Autodesk Inventor part; units mm, degrees
ref_plane "YZ Plane" through (0, 0, 0) normal (1, 0, 0) x (0, 1, 0)
ref_plane "XZ Plane" through (0, 0, 0) normal (0, 1, 0) x (-1, 0, 0)
ref_plane "XY Plane" through (0, 0, 0) normal (0, 0, 1) x (1, 0, 0)
sketch "Skizze1" plane through (0, 0, 0) normal (0, 1, 0) x (-1, 0, 0)
  line L0 (0, 0) -> (0, -54)
  line L1 (0, 0) -> (2, 0)
  line L2 (2, 0) -> (2, -10)
  line L3 (2, -10) -> (2.5, -10)
  line L4 (2.5, -10) -> (2.5, -40)
  line L5 (2.5, -40) -> (4, -40)
  line L6 (4, -40) -> (4, -44)
  line L7 (4, -44) -> (6, -44)
  line L8 (6, -44) -> (6, -48)
  line L9 (6, -48) -> (2.5, -48)
  line L10 (2.5, -48) -> (2.5, -46)
  line L11 (2.5, -46) -> (2, -46)
  line L12 (2, -46) -> (2, -54)
  line L13 (2, -54) -> (0, -54)
  point P0 (0, -27)
  point P1 (4.25, -48)
  point P2 (3.25, -40)
  point P3 (1, -54)
  point P4 (1, 0)
  dimension "d0" = 54
  dimension "d1" = 36
  dimension "d2" = 4
  dimension "d3" = 4
  dimension "d4" = 4
  dimension "d5" = 12
  dimension "d6" = 5
  dimension "d7" = 8
  dimension "d8" = 8
  dimension "d11" = 10
  dimension "d12" = 6
revolve "Umdrehung1" add sketch "Skizze1" angle 360 about axis through (0, 0, 0) along (0, 0, -1)
thread "Gewinde1"
chamfer "Fasen1" distance 0.5 angle 45 1 edges at (6, 0, -48)
chamfer "Fasen2" distance 0.5 angle 45 1 edges at (6, 0, -44)
sketch "Skizze2" plane through (0, 0, 0) normal (0, 0, 1) x (1, 0, 0)
  circle A0 centre (0, 0) radius 2
hole "Bohrung1" at (0, 0, 0) direction (0, 0, -1) diameter 3 end through all
properties part number "BRS"
Source: CAD feature listing. Evaluate the final solid. Frame: model axes, mm. A direction names the side the tool comes from. Give positions to 0.01 mm unless a question says otherwise; leave off trailing zeros. Order: outer loops, then holes, each group sorted by start corner. A loop starts at its lowest first (then second) coordinate and runs counter-clockwise, first axis right, second up. Notation, with made-up numbers: (46.5, 46.5) -> (91.5, 46.5) arc R22 ccw to (91.5, 52.5) -> close; hole circle Ø8 at (29, 5). An arc over 180 degrees is marked (long way). Use a Markdown table: item, result.
Q1. Pull-direction query (Y, two-part tool) for faces 4 (the face through (1, 2, -46)), 5 (the face through (4, -2, -44)), 6 (the face through (6, 0, -46)); classes: +Y half, -Y half, draft (parallel to the pull), parting line (faces both ways), or undercut.
A:
| item | result |
|---|---|
| face 4 | undercut |
| face 5 | draft |
| face 6 | parting line |
Q2. First-contact query: P1, Ø4, axis at y = 3.5, z = -22, coming from the -X side; P2, Ø5, axis at y = -1, z = -33, coming from the -X side; P3, Ø4, axis at x = -4, y = -1, coming from the +Z side. Flat tips, straight axial feed; report the tip coordinate or a pass-through.
A:
| item | result |
|---|---|
| P1 | x = -2 |
| P2 | x = -2.5 |
| P3 | z = -10 |
Q3. Material intervals for line 1 (Y direction, x = 0, z = -46.5); line 2 (Y direction, x = 0, z = -22); line 3 (Y direction, x = -1, z = -47.5), sorted ascending. Write a range as [from, to].
A:
| item | result |
|---|---|
| line 1 | [-6, -2.5], [-2, -1.5], [1.5, 2], [2.5, 6] |
| line 2 | [-2.5, -1.5], [1.5, 2.5] |
| line 3 | [-5.92, -2.29], [-1.73, -1.12], [1.12, 1.73], [2.29, 5.92] |
Q4. Section C-C (z = -50). Return the cut outline in (x, y).
A:
| item | result |
|---|---|
| outline | circle Ø4 at (0, 0); hole circle Ø3 at (0, 0) |
Q5. Access query for faces 1 (the face through (-0.07, 1.5, -27.38)), 2 (the face through (0.54, 2.44, -46.99)), 3 (the face through (0.54, -2.44, -25.21)). Directions: +Z, -Z, +X, -X, +Y, -Y. A direction counts if a zero-diameter tool reaches every point of the face in a straight line with its end or side. Return the directions, or none.
A:
| item | result |
|---|---|
| face 1 | +Z, -Z |
| face 2 | -Z |
| face 3 | +Z |
